from build123d import *

# Parameters (mm, degrees)
F1_DEPTH = 7.12
F2_DEPTH = 1
F3_W     = 2.36
F3_H     = 1.7178014041
F4_DEPTH = 10.791
F5_DEPTH = 25


with BuildPart() as f1:
    # F0 (on Top) → F1 (new body)
    with BuildSketch(Plane.XY):
        Polygon((0, 8), (0, 0), (10.26, 0), (14.42, 0), (22.52, 0), (27.52, 0), (27.52, 8), (22.52, 8), (14.42, 8), (1.2575370492, 8), align=None)
        Polygon((10.26, 1.2), (1.2, 1.2), (1.2575370492, 6.8), (13.0106639117, 6.8), (14.0548550674, 6.8), (14.42, 6.8), (22.52, 6.8), (26.32, 6.8), (26.32, 1.2), (22.52, 1.2), (14.42, 1.2), (13.0106639117, 1.2), align=None, mode=Mode.SUBTRACT)
        Polygon((14.0548550674, 6.8), (13.0106639117, 6.8), (13.0106639117, 1.2), (14.42, 1.2), (14.42, 6.8), align=None)
    extrude(amount=F1_DEPTH)

    # F0 (on Top) → F2 (join)
    with BuildSketch(Plane.XY):
        Polygon((0, 10.79), (0, 8), (1.2575370492, 8), (14.42, 8), (10.26, 10.79), align=None)
        Polygon((0, 8), (0, 0), (10.26, 0), (14.42, 0), (22.52, 0), (27.52, 0), (27.52, 8), (22.52, 8), (14.42, 8), (1.2575370492, 8), align=None)
        Polygon((10.26, 1.2), (1.2, 1.2), (1.2575370492, 6.8), (13.0106639117, 6.8), (14.0548550674, 6.8), (14.42, 6.8), (22.52, 6.8), (26.32, 6.8), (26.32, 1.2), (22.52, 1.2), (14.42, 1.2), (13.0106639117, 1.2), align=None, mode=Mode.SUBTRACT)
        Polygon((1.2575370492, 6.8), (1.2, 1.2), (10.26, 1.2), (13.0106639117, 1.2), (13.0106639117, 6.8), align=None)
        Polygon((14.0548550674, 6.8), (13.0106639117, 6.8), (13.0106639117, 1.2), (14.42, 1.2), (14.42, 6.8), align=None)
        Polygon((14.42, 6.8), (14.42, 1.2), (22.52, 1.2), (26.32, 1.2), (26.32, 6.8), (22.52, 6.8), align=None)
    extrude(amount=-F2_DEPTH)

    # F3 (on Front) → F4 (cut, through all)
    with BuildSketch(Plane.XZ):
        with BuildLine():
            ThreePointArc((21.5, 3.5721985959), (23.33, 1.7421985959), (25.16, 3.5721985959))
            ThreePointArc((25.16, 3.5721985959), (24.6240054096, 4.8662040054), (23.33, 5.4021985959))
            ThreePointArc((23.33, 5.4021985959), (22.0359945904, 4.8662040054), (21.5, 3.5721985959))
        make_face()
        with BuildLine():
            ThreePointArc((21.5, 3.5721985959), (22.0359945904, 4.8662040054), (23.33, 5.4021985959))
            Line((23.33, 5.4021985959), (25.16, 5.4021985959))
            Line((25.16, 5.4021985959), (25.16, 7.12))
            Line((25.16, 7.12), (21.5, 7.12))
            Line((21.5, 7.12), (21.5, 3.5721985959))
        make_face()
        with Locations((26.34, 6.2610992979)):
            Rectangle(F3_W, F3_H)
        with BuildLine():
            ThreePointArc((23.33, 5.4021985959), (24.6240054096, 4.8662040054), (25.16, 3.5721985959))
            Line((25.16, 3.5721985959), (25.16, 5.4021985959))
            Line((25.16, 5.4021985959), (23.33, 5.4021985959))
        make_face()
        with BuildLine():
            Line((27.52, -1), (27.52, 3.5302453605))
            ThreePointArc((27.52, 3.5302453605), (26.2239695669, 0.5261599489), (23.33, -1))
            Line((23.33, -1), (27.52, -1))
        make_face()
    extrude(amount=-F4_DEPTH, mode=Mode.SUBTRACT)

    # F3 (on Front) → F5 (cut)
    with BuildSketch(Plane.XZ):
        Polygon((0, 0), (4.881774541, 7.12), (0, 7.12), align=None)
    extrude(amount=-F5_DEPTH, mode=Mode.SUBTRACT)


solid = f1.part
CAD build for the part. Positions are in the model's coordinates, mm. A direction names the side the tool comes from. Coordinates: 2 decimals unless noted, no trailing zeros. Write each loop counter-clockwise with the first axis right and the second up, starting at its lowest first coordinate (ties: lowest second). Pieces come first, ordered by that corner, then holes. Notation, with made-up numbers: M 64,42.25 L 119,42.25 A34 cw 119,79.25 Z; hole C 87,65 d6. An arc over 180 degrees is marked long. Return JSON: item names as keys, results as strings.
Item 1: Slice it at D-D, the plane z = 6.5. Write the cut outline in (x, y), and give its area (3 significant figures).
Findings below:
{"outline": "M 4.46,0 L 21.5,0 L 21.5,1.2 L 14.42,1.2 L 14.42,6.8 L 21.5,6.8 L 21.5,8 L 4.46,8 L 4.46,6.8 L 13.01,6.8 L 13.01,1.2 L 4.46,1.2 Z", "area": "48.8 mm2"}
Item 2: Which spindle directions (+Z, -Z, +X, -X, +Y, -Y) get a long thin tool onto all of the face, cutting with end or side? Do faces 1 (the flat face through (26.32, 4, 3)), 2 (the flat face through (6, 9, 0)), 3 (the cylindrical face through (26.71, 3.944, 1.145)), 4 (the flat face through (13.011, 4, 4)), 5 (the flat face through (25.16, 1, 4)). Say none if no direction does.
Findings below:
{"face 1": "+Z, -Z", "face 2": "+Z, +X, -X, +Y", "face 3": "-Z, +X, +Y, -Y", "face 4": "+Z", "face 5": "+Z, +Y, -Y"}
Item 3: Two-plate mould, pull along X, no slides. Class faces 6 (the flat face through (27.52, 4, 4)), 7 (the flat face through (7, 6.8, 4)), 8 (the flat face through (13.2, 3.7, 7.12)), 9 (the flat face through (21.5, 7, 5)): +X half, -X half, draft (parallel to the pull), parting line (faces both ways), or undercut.
Findings below:
{"face 6": "+X half", "face 7": "undercut", "face 8": "draft", "face 9": "undercut"}
Item 4: Probe line 1 (Y direction, x = 19.75, z = 5.75); line 2 (X direction, y = 1.75, z = 3.5); line 3 (Z direction, x = 6.25, y = 8.5). List the from-to ranges inside material, lowest first. Write a range as from..to.
Findings below:
{"line 1": "y = 0..1.2, 6.8..8", "line 2": "x = 13.01..14.42, 26.32..27.52", "line 3": "z = -1..0"}
Item 5: Drop flat-ended pins along their axis: pin 1 Ø1.3 at (y, z) = (0.5, 4.5) entering from -X; pin 2 Ø4 at (y, z) = (4.5, 1.5) entering from +X; pin 3 Ø2 at (y, z) = (1.5, 5.5) entering from -X. Give the stop position or say it passes through.
Findings below:
{"pin 1": "stops at x = 2.64", "pin 2": "stops at x = 27.52", "pin 3": "stops at x = 3.12"}
Item 6: Slice it at C-C, the plane x = 8. Write the cut outline in (y, z).
Findings below:
{"outline": "M 0,-1 L 10.79,-1 L 10.79,0 L 8,0 L 8,7.12 L 6.8,7.12 L 6.8,0 L 1.2,0 L 1.2,7.12 L 0,7.12 Z"}
Item 7: Slice it at A-A, the plane y = 5. Write the cut outline in (x, z), and give its area (3 significant figures).
Findings below:
{"outline": "M 0,-1 L 23.33,-1 A4.92 ccw 25.65,0 L 14.42,0 L 14.42,7.12 L 13.01,7.12 L 13.01,0 L 1.24,0 L 1.24,1.81 L 0,0 Z; M 26.32,0.63 A4.92 ccw 27.52,3.53 L 27.52,5.4 L 26.32,5.4 Z", "area": "40.5 mm2"}
Item 8: Slice it at B-B, the plane y = 0.5. Write the cut outline in (x, z).
Findings below:
{"outline": "M 0,-1 L 23.33,-1 A4.92 ccw 27.52,3.53 L 27.52,5.4 L 25.16,5.4 L 25.16,3.57 A1.83 cw 21.5,3.57 L 21.5,7.12 L 4.88,7.12 L 0,0 Z"}
